from build123d import *

# Parameters (mm, degrees)
CHAMFER1_SIZE = 0.5


with BuildPart() as part:
    # Sketch1 → Revolve1 (revolve)
    with BuildSketch(Plane.XY):
        Polygon((0, 4.7875), (0, 7), (-2, 7), (-2, 0), (29.237, 0), (29.237, 4.7875), (27.737, 4.7875), (27.737, 4.47), (27, 4.47), (27, 4.7875), align=None)
    revolve(axis=Axis((-78.535413295, 0, 0), (1, 0, 0)))

    # Chamfer1
    chamfer1_edges = [part.edges().sort_by_distance(p)[0] for p in [
        (0, -4.7875, 0),
        (-2, -7, 0),
        (29.237, -4.7875, 0),
    ]]
    chamfer(chamfer1_edges, length=CHAMFER1_SIZE)


solid = part.part
The listing builds one solid part. Answer for the finished solid, in the listing's coordinates (mm). A direction names the side the tool comes from. Coordinates: 2 decimals unless noted, no trailing zeros. Order: outer loops, then holes, each group sorted by start corner. A loop starts at its lowest first (then second) coordinate and runs counter-clockwise, first axis right, second up.
Q1. Consider line 1 (X direction, y = 0, z = -5.5); line 2 (Y direction, x = 24, z = -2); line 3 (Z direction, x = 3, y = -1.75). Determine where each line is inside the solid, lowest interval first.
Q2. A cutting plane is placed at A-A, the plane z = 0. Write down the section's boundary in (x, y).
Q3. Which of the six approach directions +Z, -Z, +X, -X, +Y, -Y give full straight-line access (tool end or side, diameter ignored) to faces 4 (the face through (-0.76, 6.466, -2.681)), 5 (the face through (13.56, -3.8, -2.91))?
Q4. A cutting plane is placed at C-C, the plane x = 24. Write down the section's boundary in (y, z) (1 decimal).
Q5. Given P1, Ø2, axis at x = 2, y = -2, coming from the +Z side; P2, Ø8, axis at x = 11, z = -2, coming from the -Y side; P3, Ø1, axis at x = 24, y = 2, coming from the +Z side, each flat-ended and moving along its own axis, determine where each tip first touches the part or whether it passes through.
Q6. For a pull along X with two mould halves and no side action, classify faces 1 (the face through (27.363, -0.969, -4.364)), 2 (the face through (28.23, -3.8, -2.91)), 3 (the face through (29.237, 0, 0)) as pulls with the +X half, pulls with the -X half, needs draft (parallel to the pull), parting line crosses it, or undercut.
Answers follow:
1. line 1: x = -2 to 0
1. line 2: y = -4.35 to 4.35
1. line 3: z = -4.46 to 4.46
2. outline: (-2, -6.5) - (-1.5, -7) - (0, -7) - (0, -5.29) - (0.5, -4.79) - (27, -4.79) - (27, -4.47) - (27.74, -4.47) - (27.74, -4.79) - (28.74, -4.79) - (29.24, -4.29) - (29.24, 4.29) - (28.74, 4.79) - (27.74, 4.79) - (27.74, 4.47) - (27, 4.47) - (27, 4.79) - (0.5, 4.79) - (0, 5.29) - (0, 7) - (-1.5, 7) - (-2, 6.5) - close
3. face 4: +X, -X
3. face 5: +X
4. outline: circle Ø9.6 at (0, 0)
5. P1: stops at z = 4.68
5. P2: stops at y = -4.79
5. P3: stops at z = 4.55
6. face 1: undercut
6. face 2: needs draft
6. face 3: pulls with the +X half
